Input: part model. Units: mm. Frame: model coordinates. A direction names the side the tool comes from. Round coordinates to 2 decimals unless told otherwise and drop trailing zeros. Write each loop counter-clockwise with the first axis right and the second up, starting at its lowest first coordinate (ties: lowest second). Pieces come first, ordered by that corner, then holes. Notation, with made-up numbers: (-23.5, 0.25) - (3.5, 0.25) arc R23 ccw to (3.5, 9.25) - close; hole circle Ø4 at (53, -15.75). An arc over 180 degrees is marked (long way). Use one line per item in the form item = value.
```python
from build123d import *

# Parameters (mm, degrees)
F0_R          = 25.4
F0_R_2        = 7.62
F1_DEPTH      = 127
F0_R_3        = 22.86
F2_DEPTH      = 101.6
F4_DEPTH      = 17.78
F4_DEPTH_BACK = 17.78
F5_W          = 60.96
F5_H          = 60.96
F6_DEPTH      = 25.4
F6_DEPTH_BACK = 25.4
F7_R          = 5.08
F8_T4_ANGLE   = 315.8495903275
F8_T13_ANGLE  = 315.8495903275
F9_R          = 27.94
F9_R_2        = 22.86
F10_DEPTH     = 12.7
F11_SIZE      = 2.54


# Not quite as in the source:
# - a fillet or chamfer that OpenCascade refuses, or shapes differently, is made with other operations: its cross-section is extruded or revolved along the edge and cut away or added


with BuildPart() as f1:
    # F0 (on Top) → F1 (new body)
    with BuildSketch(Plane.XY):
        Circle(F0_R)
        Circle(F0_R_2, mode=Mode.SUBTRACT)
    extrude(amount=F1_DEPTH)



with BuildPart() as f2:
    # F0 (on Top) → F2 (new body)
    with BuildSketch(Plane.XY):
        with Locations((101.6, 0)):
            Circle(F0_R_3)
        with Locations((101.6, 0)):
            Circle(F0_R_2, mode=Mode.SUBTRACT)
    extrude(amount=F2_DEPTH)


with BuildPart() as f1_1:
    add(f1.part)

    add(f2.part)  # F4 merges F2
    # F3 (on Front) → F4 (join, two sides)
    with BuildSketch(Plane.XZ) as f4_sk:
        with BuildLine():
            Line((20.32, 127), (20.32, 0))
            Line((20.32, 0), (81.28, 0))
            Line((81.28, 0), (81.28, 81.28))
            ThreePointArc((81.28, 81.28), (61.5844056789, 108.82076155), (33.02, 127))
            Line((33.02, 127), (20.32, 127))
        make_face()
        with BuildLine():
            Line((33.02, 50.4039023765), (33.02, 113.9039023765))
            ThreePointArc((33.02, 113.9039023765), (55.7015227305, 97.7137904926), (71.12, 74.5008252602))
            Line((71.12, 74.5008252602), (71.12, 50.4039023765))
            Line((71.12, 50.4039023765), (33.02, 50.4039023765))
        make_face(mode=Mode.SUBTRACT)
    extrude(amount=F4_DEPTH)
    extrude(f4_sk.sketch, amount=-F4_DEPTH_BACK)

    # F5 (on Front) → F6 (cut, two sides)
    with BuildSketch(Plane.XZ) as f6_sk:
        with Locations((-2.54, 55.88)):
            Rectangle(F5_W, F5_H)
    extrude(amount=F6_DEPTH, mode=Mode.SUBTRACT)
    extrude(f6_sk.sketch, amount=-F6_DEPTH_BACK, mode=Mode.SUBTRACT)

    # F7
    f7_edges = [f1_1.edges().sort_by_distance(p)[0] for p in [
        (33.02, 0, 113.903902),
        (33.02, 0, 50.403902),
        (71.12, 0, 50.403902),
        (71.12, 0, 74.500825),
    ]]
    fillet(f7_edges, radius=F7_R)

    # F8: chamfer of 2.54 on 4 edges, made by hand


with BuildPart() as f8_tool2:
    # F8_s3 → F8_t4 (revolve)
    with BuildSketch(Plane(origin=(0, 0, 0), x_dir=(0, 0, 1), z_dir=(0.3758232659, -0.9266913579, 0))):
        Polygon((0, -22.86), (2.54, -25.4), (0, -25.4), align=None)
    revolve(axis=Axis((0, 0, 0), (0, 0, 1)), revolution_arc=F8_T4_ANGLE)

    split(bisect_by=Plane.YZ.offset(20.32), keep=Keep.BOTTOM)


with BuildPart() as f1_2:
    add(f1_1.part)

    # F8_t1: cut F8_tool2
    add(f8_tool2.part, mode=Mode.SUBTRACT)

    # F8_s6 → F8_t7 (revolve, cut)
    with BuildSketch(Plane.XZ):
        Polygon((10.16, 25.4), (7.62, 22.86), (7.62, 25.4), align=None)
    revolve(axis=Axis((0, 0, 25.4), (0, 0, -1)), mode=Mode.SUBTRACT)

    # F8_s8 → F8_t9 (revolve, cut)
    with BuildSketch(Plane.XZ):
        Polygon((10.16, 86.36), (7.62, 88.9), (7.62, 86.36), align=None)
    revolve(axis=Axis((0, 0, 86.36), (0, 0, -1)), mode=Mode.SUBTRACT)


with BuildPart() as f8_tool11:
    # F8_s12 → F8_t13 (revolve)
    with BuildSketch(Plane(origin=(0, 0, 0), x_dir=(0, 0, 1), z_dir=(0.3758232659, -0.9266913579, 0))):
        Polygon((127, -22.86), (124.46, -25.4), (127, -25.4), align=None)
    revolve(axis=Axis((0, 0, 127), (0, 0, 1)), revolution_arc=F8_T13_ANGLE)

    split(bisect_by=Plane.YZ.offset(20.32), keep=Keep.BOTTOM)


with BuildPart() as f1_3:
    add(f1_2.part)

    # F8_t10: cut F8_tool11
    add(f8_tool11.part, mode=Mode.SUBTRACT)

    # F9 (on Top) → F10 (join)
    with BuildSketch(Plane.XY):
        with Locations((101.6, 0)):
            Circle(F9_R)
        with Locations((101.6, 0)):
            Circle(F9_R_2, mode=Mode.SUBTRACT)
    extrude(amount=F10_DEPTH)

    # F11
    f11_edges = [f1_3.edges().sort_by_distance(p)[0] for p in [
        (129.54, 0, 0),
        (129.54, 0, 12.7),
        (78.74, 0, 101.6),
        (93.98, 0, 101.6),
        (-7.62, 0, 127),
    ]]
    chamfer(f11_edges, length=F11_SIZE)


solid = f1_3.part
```
(1) Cut plane C-C on x = 101.6. Output: boundary loops of the cut face in (y, z), then the cut area to 3 significant figures.
Derived:
outline = (-27.94, 2.54) - (-25.4, 0) - (-7.62, 0) - (-7.62, 99.06) - (-10.16, 101.6) - (-20.32, 101.6) - (-22.86, 99.06) - (-22.86, 12.7) - (-25.4, 12.7) - (-27.94, 10.16) - close; (7.62, 0) - (25.4, 0) - (27.94, 2.54) - (27.94, 10.16) - (25.4, 12.7) - (22.86, 12.7) - (22.86, 99.06) - (20.32, 101.6) - (10.16, 101.6) - (7.62, 99.06) - close
area = 3,200 mm^2
(2) Access query for faces 5 (the face through (51, 0, 0)), 6 (the face through (71.12, 0, 65)), 7 (the face through (-6.14, 4.71, 88.78)). Directions: +Z, -Z, +X, -X, +Y, -Y. A direction counts if a zero-diameter tool reaches every point of the face in a straight line with its end or side. Return the directions, or none.
Derived:
face_5 = -Z, +X, -X, +Y, -Y
face_6 = +Y, -Y
face_7 = none
(3) Cut plane B-B on x = 0. Output: boundary loops of the cut face in (y, z).
Derived:
outline = (-25.4, 2.54) - (-22.86, 0) - (-7.62, 0) - (-7.62, 22.86) - (-10.16, 25.4) - (-25.4, 25.4) - close; (-25.4, 86.36) - (-10.16, 86.36) - (-7.62, 88.9) - (-7.62, 124.46) - (-10.16, 127) - (-22.86, 127) - (-25.4, 124.46) - close; (7.62, 0) - (22.86, 0) - (25.4, 2.54) - (25.4, 25.4) - (10.16, 25.4) - (7.62, 22.86) - close; (7.62, 88.9) - (10.16, 86.36) - (25.4, 86.36) - (25.4, 124.46) - (22.86, 127) - (10.16, 127) - (7.62, 124.46) - close
(4) Cut plane A-A on z = 41. Output: boundary loops of the cut face in (x, y).
Derived:
outline = (27.94, -17.78) - (81.28, -17.78) - (81.28, -10.47) arc R22.86 ccw (long way) to (81.28, 10.47) - (81.28, 17.78) - (27.94, 17.78) - close; hole circle Ø15.24 at (101.6, 0)
(5) Material intervals for L1, parallel to Y at x = 101, z = 74; L2, parallel to Z at x = 12, y = 10.5; L3, parallel to X at y = -14.5, z = 52.5, sorted ascending.
Derived:
L1 = -22.85 to -7.6, 7.6 to 22.85
L2 = 0 to 25.4, 86.36 to 127
L3 = 27.94 to 33.99, 70.15 to 81.28, 83.93 to 119.27
(6) Draft query along Z for faces 1 (the face through (27.94, 0, 55)), 2 (the face through (124.4, 3.9, 12.7)), 3 (the face through (51, -17.78, 50)), 4 (the face through (1, 11, 86.36)). Return one class per face: released by +Z, released by -Z, zero draft, split by the parting line, or undercut.
Derived:
face_1 = undercut
face_2 = released by +Z
face_3 = zero draft
face_4 = undercut
(7) First-contact query: pin 1 Ø2 at (y, z) = (14.5, 47.5) entering from +X; pin 2 Ø3 at (x, y) = (95, -3) entering from +Z; pin 3 Ø2 at (y, z) = (-15.5, 61.5) entering from +X. Flat tips, straight axial feed; report the tip coordinate or a pass-through.
Derived:
pin_1 = 120.05
pin_2 = 100.19
pin_3 = 119.27
(8) Cut plane D-D on y = 2. Count the separate pieces of the cut face and the enclosed holes in it, then the cut area to 3 significant figures.
Derived:
separate_pieces = 4
enclosed_holes = 1
area = 9,630 mm^2
